from build123d import *

# Parameters (mm, degrees)
BASPROSKE_W        = 6.35
BASPROSKE_H        = 15.24
TOOTHCUT_DEPTH     = 23.468593636
TEETHCUTS_COUNT    = 10
TEETHCUTS_ANGLE    = 324
BORSKE_R           = 0.396875
BORE_DEPTH         = 50.8000508
KEYSKE_W           = 0.254
KEYSKE_H           = 0.619125
KEYWAY_DEPTH       = 50.8000508
SKETCH1_R          = 3.175
CUT_EXTRUDE1_DEPTH = 23.027224313


with BuildPart() as part:
    # BasProSke → Base-Revolve (revolve)
    with BuildSketch(Plane(origin=(0, 0, 0), x_dir=(1, 0, 0), z_dir=(0, 1, 0)), mode=Mode.PRIVATE) as base_revolve_sk:
        with Locations((3.175, 7.62)):
            Rectangle(BASPROSKE_W, BASPROSKE_H)
    revolve(base_revolve_sk.sketch.rotate(Axis((-10, 0, 0), (1, 0, 0)), 180), axis=Axis((-10, 0, 0), (1, 0, 0)))

    # TooCutSke → ToothCut (cut, through all)
    with BuildSketch(Plane(origin=(0, 0, 0), x_dir=(0, 0, -1), z_dir=(1, 0, 0))):
        with BuildLine():
            ThreePointArc((1.512171166, 9.402912925), (0, 9.52373), (-1.512171166, 9.402912925))
            ThreePointArc((-1.512171166, 9.402912925), (-2.144739364, 12.480481638), (-4.466452315, 14.597371026))
            ThreePointArc((-4.466452315, 14.597371026), (0, 15.2654), (4.466452315, 14.597371026))
            ThreePointArc((4.466452315, 14.597371026), (2.144739364, 12.480481638), (1.512171166, 9.402912925))
        make_face()
    toothcut = extrude(amount=TOOTHCUT_DEPTH, mode=Mode.SUBTRACT)

    # TeethCuts: ToothCut ×10 about axis
    teethcuts_axis = Axis((-10, 0, 0), (1, 0, 0))
    for i in range(1, TEETHCUTS_COUNT):
        add(toothcut.rotate(teethcuts_axis, i * TEETHCUTS_ANGLE / (TEETHCUTS_COUNT - 1)), mode=Mode.SUBTRACT)

    # BorSke → Bore (cut, symmetric)
    with BuildSketch(Plane(origin=(0, 0, 0), x_dir=(0, 0, -1), z_dir=(1, 0, 0))):
        with Locations(Location((0, 0, 0), (0, 0, 180))):
            Circle(BORSKE_R)
    extrude(amount=BORE_DEPTH, both=True, mode=Mode.SUBTRACT)

    # KeySke → Keyway (cut, symmetric)
    with BuildSketch(Plane(origin=(0, 0, 0), x_dir=(0, 0, -1), z_dir=(1, 0, 0))):
        with Locations((0, 0.3095625)):
            Rectangle(KEYSKE_W, KEYSKE_H)
    extrude(amount=KEYWAY_DEPTH, both=True, mode=Mode.SUBTRACT)

    # Sketch1 → Cut-Extrude1 (cut, through all)
    with BuildSketch(Plane.ZY):
        Circle(SKETCH1_R)
    extrude(amount=-CUT_EXTRUDE1_DEPTH, mode=Mode.SUBTRACT)


solid = part.part
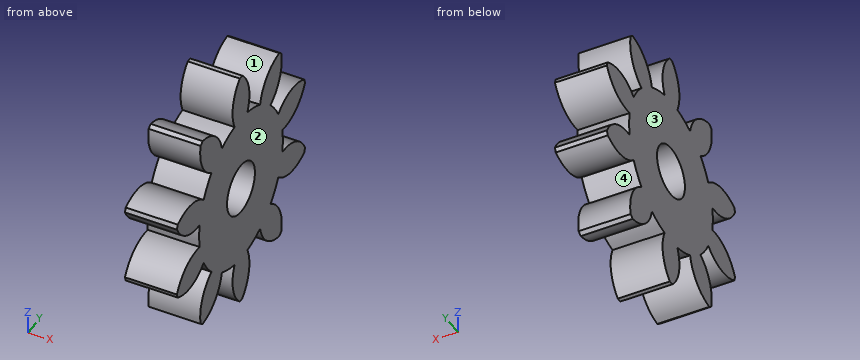
Verification items for the finished model (mm, model axes). Face numbers are marked on the shaded views. A direction names the side the tool comes from. Coordinates: 2 decimals unless noted, no trailing zeros. Order: outer loops, then holes, each group sorted by start corner. A loop starts at its lowest first (then second) coordinate and runs counter-clockwise, first axis right, second up. Notation, with made-up numbers: M -14.5,-14 L 13.5,-14 A17 ccw 13.5,9 Z; hole C 71,-31.5 d3. An arc over 180 degrees is marked long. Return JSON: item names as keys, results as strings.
1) Thickness scan on L1, parallel to Y at x = 1, z = -10; L2, parallel to Y at x = 4.5, z = 0 (3 decimals); L3, parallel to Y at x = 0.5, z = -12. Record the ranges inside material, lowest first. Write a range as [from, to].
Answer list:
{"L1": "[-9.15, -4.92], [-1.69, 1.69], [4.92, 9.15]", "L2": "[-9.524, -3.175], [3.175, 9.524]", "L3": "[-9.22, -7.05], [-1.9, 1.9], [7.05, 9.22]"}
2) Access from +Z, -Z, +X, -X, +Y, -Y to the whole of each face (thin tool, end or side, straight path). Record for the marked faces 1 and 2.
Answer list:
{"face 1": "+Z, +X, -X", "face 2": "+Z, -Z, +X, +Y, -Y"}
3) Cross-section at D-D, the plane y = -5.5. Record the boundary of the cut face in (x, z), and give its area (3 significant figures).
Answer list:
{"outline": "M 0,-10.8 L 6.35,-10.8 L 6.35,10.8 L 0,10.8 Z", "area": "137 mm2"}
4) Cross-section at B-B, the plane z = 11.5. Record the boundary of the cut face in (x, y).
Answer list:
{"outline": "M 0,-9.28 L 6.35,-9.28 L 6.35,-6.25 L 0,-6.25 Z; M 0,-1.92 L 6.35,-1.92 L 6.35,1.92 L 0,1.92 Z; M 0,6.25 L 6.35,6.25 L 6.35,9.28 L 0,9.28 Z"}
5) Cross-section at A-A, the plane z = 0. Record the boundary of the cut face in (x, y) (3 decimals), and give its area (3 significant figures).
Answer list:
{"outline": "M 0,-9.524 L 6.35,-9.524 L 6.35,-3.175 L 0,-3.175 Z; M 0,3.175 L 6.35,3.175 L 6.35,9.524 L 0,9.524 Z", "area": "80.6 mm2"}
6) Cross-section at C-C, the plane z = -9. Record the boundary of the cut face in (x, y).
Answer list:
{"outline": "M 0,-8.8 L 6.35,-8.8 L 6.35,-4.48 L 0,-4.48 Z; M 0,-3.11 L 6.35,-3.11 L 6.35,3.11 L 0,3.11 Z; M 0,4.48 L 6.35,4.48 L 6.35,8.8 L 0,8.8 Z"}
7) Release check for a two-part mould opening along Y. For the marked faces 3 and 4 record: +Y half, -Y half, draft (parallel to the pull), parting line (faces both ways), or undercut.
Answer list:
{"face 3": "draft", "face 4": "undercut"}
8) Gauge pin test, flat end, axial feed: pin 1 (2 mm diameter, centred on x = 2.5, y = -9, fed in from -Z). Record the tip position at first contact, or that the pin passes through.
Answer list:
{"pin 1": "z = -12.5"}
